Read the model definition and answer for the solid it produces. Units are mm, in the model's axes. Round coordinates to 2 decimals unless told otherwise and drop trailing zeros. Order: outer loops, then holes, each group sorted by start corner. A loop starts at its lowest first (then second) coordinate and runs counter-clockwise, first axis right, second up.
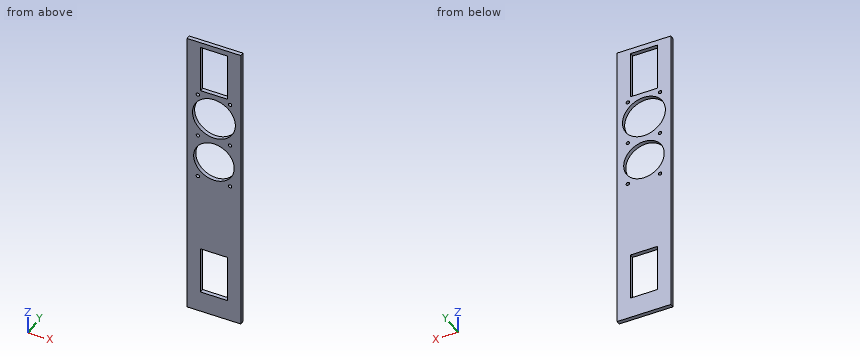
Autodesk Inventor part; units mm, degrees
ref_plane "YZ Plane" through (0, 0, 0) normal (1, 0, 0) x (0, 1, 0)
ref_plane "XZ Plane" through (0, 0, 0) normal (0, 1, 0) x (-1, 0, 0)
ref_plane "XY Plane" through (0, 0, 0) normal (0, 0, 1) x (1, 0, 0)
sketch "Sketch1" plane through (0, 0, 0) normal (0, 1, 0) x (-1, 0, 0)
  line L0 (-31.75, -177.8) -> (31.75, -177.8)
  line L1 (31.75, -177.8) -> (31.75, 177.8)
  line L2 (31.75, 177.8) -> (-31.75, 177.8)
  line L3 (-31.75, 177.8) -> (-31.75, -177.8)
  line L4 (-31.75, -177.8) -> (31.75, 177.8) construction
  line L5 (31.75, -177.8) -> (-31.75, 177.8) construction
  line L6 (15.875, -152.4) -> (-15.875, -152.4)
  line L7 (-15.875, -152.4) -> (-15.875, -95.25)
  line L8 (-15.875, -95.25) -> (15.875, -95.25)
  line L9 (15.875, -95.25) -> (15.875, -152.4)
  line L10 (-15.875, 171.45) -> (15.875, 171.45)
  line L11 (15.875, 171.45) -> (15.875, 114.3)
  line L12 (15.875, 114.3) -> (-15.875, 114.3)
  line L13 (-15.875, 114.3) -> (-15.875, 171.45)
  point P0 (0, 0)
  point P1 (0, -95.25)
  point P2 (0, 114.3)
  dimension "d0" = 31.75
  dimension "d1" = 57.15
  dimension "d2" = 355.6
  dimension "d3" = 25.4
  dimension "d4" = 63.5
  dimension "d6" = 6.35
extrude "Plate1" add sketch "Sketch1" along normal blind 4.7625
sketch "Sketch2" plane through (0, 4.7625, 0) normal (0, 1, 0) x (1, 0, 0)
  circle A0 centre (0, -82.55) radius 25.4
  circle A1 centre (0, -25.4) radius 24.0284
  point P0 (0, 0)
  dimension "d7" = 50.8
  dimension "d8" = 82.55
  dimension "d9" = 48.0568
  dimension "d10" = 57.15
extrude "Cut1" cut sketch "Sketch2" against normal blind 4.7625
sketch "Sketch3" plane through (0, 4.7625, 0) normal (0, 1, 0) x (1, 0, 0)
  line L0 (31.75, 177.8) -> (31.75, -177.8) construction
  line L1 (31.75, -177.8) -> (-31.75, -177.8) construction
  circle A0 centre (0, -82.55) radius 25.4
  point P0 (0, 0)
  point P1 (19.05, -107.95)
  point P2 (-19.05, -107.95)
  point P3 (19.05, -53.975)
  point P4 (-19.05, -53.975)
  point P5 (19.05, 0)
  point P6 (-19.05, 0)
  dimension "d13" = 12.7
  dimension "d16" = 38.1
  dimension "d19" = 53.975
  dimension "d22" = 28.575
hole "Hole1" at (19.05, 4.7625, 107.95) at (-19.05, 4.7625, 107.95) at (19.05, 4.7625, 53.975) at (-19.05, 4.7625, 53.975) at (19.05, 4.7625, 0) at (-19.05, 4.7625, 0) direction (0, -1, 0) diameter 3.9624 end through all
equation "\"d11\" = Thickness"
equation "\"d28\" = Thickness"
equation "\"d5\" = Thickness"
equation "\"BendRadius\" = Thickness"
equation "\"BendReliefWidth\" = Thickness"
equation "\"BendReliefDepth\" = 0.5 * Thickness"
equation "\"CornerReliefSize\" = 4 * Thickness"
equation "\"MinimumRemnant\" = 2 * Thickness"
equation "\"TransitionRadius\" = BendRadius"
equation "\"JacobiRadiusSize\" = BendRadius"
equation "\"GapSize\" = Thickness"
properties part number "PLATE,FRONT" material "Aluminum 6061"
Q1. A cutting plane is placed at B-B, the plane z = 82.55. Give the vertices of the cut face in (x, y).
Outcome:
outline: (-31.75, 0) - (-25.4, 0) - (-25.4, 4.76) - (-31.75, 4.76) - close; (25.4, 0) - (31.75, 0) - (31.75, 4.76) - (25.4, 4.76) - close
Q2. A flat-ended cylindrical pin translates along its axis: pin 1 (4.5 mm diameter, centred on x = 19.05, z = 0, fed in from -Y). Find the tip coordinate at first contact, or state that the pin passes through.
Outcome:
pin 1: stops at y = 0
Q3. Straight lines are drawn through the part: probe 1 along Z at (x, y) = (0, 3.8); probe 2 along X at (y, z) = (3.4, 53.5); probe 3 along X at (y, z) = (3.9, 136) (3 decimals). For each, find the intervals that lie inside material, in ascending order.
Outcome:
probe 1: z = -177.8 to -152.4, -95.25 to 1.37, 49.43 to 57.15, 107.95 to 114.3, 171.45 to 177.8
probe 2: x = -31.75 to -20.97, -17.13 to 17.13, 20.97 to 31.75
probe 3: x = -31.75 to -15.875, 15.875 to 31.75
Q4. A cutting plane is placed at A-A, the plane x = 0. Give the vertices of the cut face in (y, z), plus the area to 3 significant figures.
Outcome:
outline: (0, -177.8) - (4.76, -177.8) - (4.76, -152.4) - (0, -152.4) - close; (0, -95.25) - (4.76, -95.25) - (4.76, 1.37) - (0, 1.37) - close; (0, 49.43) - (4.76, 49.43) - (4.76, 57.15) - (0, 57.15) - close; (0, 107.95) - (4.76, 107.95) - (4.76, 114.3) - (0, 114.3) - close; (0, 171.45) - (4.76, 171.45) - (4.76, 177.8) - (0, 177.8) - close
area: 678 mm2
Q5. A cutting plane is placed at C-C, the plane y = 2.2. Give the number of separate pieces and of enclosed holes in the cut face, plus the area to 3 significant figures.
Outcome:
separate pieces: 1
enclosed holes: 10
area: 15,000 mm2
